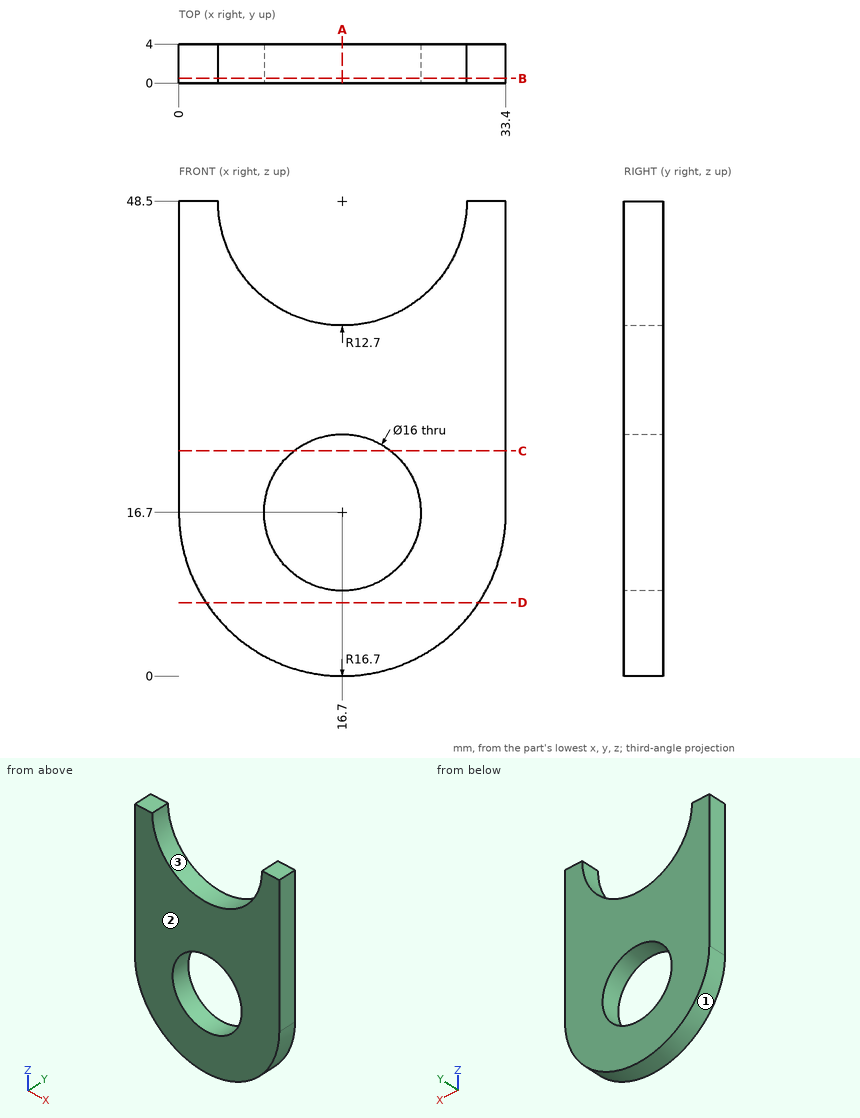
Input: dimensioned drawing with shaded views. Units: mm. Origin: part minimum x, y, z. Coordinates: 2 decimals unless noted, no trailing zeros. Loops run counter-clockwise (first coordinate to the right, second up) from the corner with the lowest first, then second, coordinate; pieces in that order, holes last. Notation, with made-up numbers: (-35, 45) -> (-13, 45) arc R16 cw to (-13, 54) -> close; hole circle Ø7 at (-25.5, 0.5). An arc over 180 degrees is marked (long way). Use a Markdown table: item, result. Add a question column.
(1) Mould query, pull axis X, two halves, no side actions, for the marked faces 1, 2 and 3. Classes: pulls with the +X half, pulls with the -X half, needs draft (parallel to the pull), parting line crosses it, or undercut.
(2) Section query B-B, the plane y = 0.5. Return loops of the section in (x, z), plus the area to 3 significant figures.
(3) Line query: line 1 along X through (y, z) = (2.55, 16.7); line 2 along Z through (x, y) = (16.5, 2.95); line 3 along X through (y, z) = (1.95, 23). Output: solid intervals per line, ascending.
(4) Pin query (flat end, axial travel): pin 1 Ø1.5 at (y, z) = (3.5, 10.5) entering from +X; pin 2 Ø2 at (x, y) = (15, 2) entering from +Z; pin 3 Ø1 at (x, y) = (26, 1) entering from -Z. Return the tip coordinate at first contact, or that it passes through.
(5) Section query C-C, the plane z = 23. Return loops of the section in (x, y), plus the area to 3 significant figures.
(6) Section query D-D, the plane z = 7.5. Return loops of the section in (x, y), plus the area to 3 significant figures.
(7) Section query A-A, the plane x = 16.7. Return loops of the section in (y, z).
Answer:
| question | item | result |
|---|---|---|
| 1 | face 1 | parting line crosses it |
| 1 | face 2 | needs draft |
| 1 | face 3 | undercut |
| 2 | outline | (0, 16.7) arc R16.7 ccw to (33.4, 16.7) -> (33.4, 48.5) -> (29.4, 48.5) arc R12.7 cw to (4, 48.5) -> (0, 48.5) -> close; hole circle Ø16 at (16.7, 16.7) |
| 2 | area | 1,050 mm^2 |
| 3 | line 1 | x = 0 to 8.7, 24.7 to 33.4 |
| 3 | line 2 | z = 0 to 8.7, 24.7 to 35.8 |
| 3 | line 3 | x = 0 to 11.77, 21.63 to 33.4 |
| 4 | pin 1 | stops at x = 32.49 |
| 4 | pin 2 | stops at z = 36.09 |
| 4 | pin 3 | stops at z = 2.51 |
| 5 | outline | (0, 0) -> (11.77, 0) -> (11.77, 4) -> (0, 4) -> close; (21.63, 0) -> (33.4, 0) -> (33.4, 4) -> (21.63, 4) -> close |
| 5 | area | 94.2 mm^2 |
| 6 | outline | (2.76, 0) -> (30.64, 0) -> (30.64, 4) -> (2.76, 4) -> close |
| 6 | area | 111 mm^2 |
| 7 | outline | (0, 0) -> (4, 0) -> (4, 8.7) -> (0, 8.7) -> close; (0, 24.7) -> (4, 24.7) -> (4, 35.8) -> (0, 35.8) -> close |
